Read the model definition and answer for the solid it produces. Units are mm, in the model's axes. Coordinates: 2 decimals unless noted, no trailing zeros. Write each loop counter-clockwise with the first axis right and the second up, starting at its lowest first coordinate (ties: lowest second). Pieces come first, ordered by that corner, then holes. Notation, with made-up numbers: (-34.75, -1) -> (-19.75, -1) arc R29 cw to (-19.75, 35) -> close; hole circle Ø5 at (-37, -23). An arc over 180 degrees is marked (long way). Use CSV: the item, a comma, the result in double quotes.
from build123d import *

# Parameters (mm, degrees)
ESQUISSE1_W                  = 1700
ESQUISSE1_H                  = 150
BOSS_EXTRU_1_DEPTH           = 25
ENL_V_MAT_EXTRU_1_DEPTH      = 1707.78791887
ENL_V_MAT_EXTRU_1_DEPTH_BACK = 1707.78791887
CHANFREIN2_SIZE              = 40
CHANFREIN3_SIZE              = 5


with BuildPart() as part:
    # Esquisse1 → Boss.-Extru.1 (new body)
    with BuildSketch(Plane.XY):
        with Locations((850, 75)):
            Rectangle(ESQUISSE1_W, ESQUISSE1_H)
    extrude(amount=BOSS_EXTRU_1_DEPTH)

    # Esquisse2 → Enlèv. mat.-Extru.1 (cut, two sides: drawn at the far end of the back side and taken through both)
    with BuildSketch(Plane(origin=(0, 150, 0), x_dir=(1, 0, 0), z_dir=(0, 1, 0)).offset(-ENL_V_MAT_EXTRU_1_DEPTH_BACK)):
        Polygon((100, 0), (101.227845609, -10), (61.227845609, -10), (62.455691218, 0), align=None)
        Polygon((1637.544308782, 0), (1638.772154391, -10), (1598.772154391, -10), (1600, 0), align=None)
        Polygon((868.772154391, 0), (831.227845609, 0), (830, -10), (870, -10), align=None)
    extrude(amount=ENL_V_MAT_EXTRU_1_DEPTH + ENL_V_MAT_EXTRU_1_DEPTH_BACK, mode=Mode.SUBTRACT)

    # Chanfrein2
    chanfrein2_edges = [part.edges().sort_by_distance(p)[0] for p in [
        (1700, 0, 12.5),
        (0, 0, 12.5),
    ]]
    chamfer(chanfrein2_edges, length=CHANFREIN2_SIZE)

    # Chanfrein3
    chanfrein3_edges = [part.edges().sort_by_distance(p)[0] for p in [
        (850, 150, 25),
        (0, 95, 25),
        (850, 0, 25),
        (1700, 95, 25),
        (1680, 20, 25),
        (20, 20, 25),
    ]]
    chamfer(chanfrein3_edges, length=CHANFREIN3_SIZE)


solid = part.part
1. A cutting plane is placed at A-A (y = 94.5). Give the vertices of the cut face in (x, z), and give its area (3 significant figures).
Solutions:
outline,"(0, 0) -> (62.46, 0) -> (61.23, 10) -> (101.23, 10) -> (100, 0) -> (831.23, 0) -> (830, 10) -> (870, 10) -> (868.77, 0) -> (1600, 0) -> (1598.77, 10) -> (1638.77, 10) -> (1637.54, 0) -> (1700, 0) -> (1700, 20) -> (1695, 25) -> (5, 25) -> (0, 20) -> close"
area,"41,300 mm^2"
2. This flat-tipped pin is pushed along its axis until it touches: pin 1 Ø1.5 at (x, z) = (447.5, 21.5) entering from -Y. Where does it stop, or does it pass through?
Solutions:
pin 1,"stops at y = 0.75"
3. A cutting plane is placed at B-B (y = 21). Give the vertices of the cut face in (x, z), and give its area (3 significant figures).
Solutions:
outline,"(19, 0) -> (62.46, 0) -> (61.23, 10) -> (101.23, 10) -> (100, 0) -> (831.23, 0) -> (830, 10) -> (870, 10) -> (868.77, 0) -> (1600, 0) -> (1598.77, 10) -> (1638.77, 10) -> (1637.54, 0) -> (1681, 0) -> (1681, 20) -> (1673.93, 25) -> (26.07, 25) -> (19, 20) -> close"
area,"40,400 mm^2"
4. Find the intervals of material crossed by line 1 along X through (y, z) = (65, 1.5); line 2 along X through (y, z) = (31, 5.75); line 3 along Z through (x, y) = (838, 50), in increasing order.
Solutions:
line 1,"x = 0 to 62.27, 100.18 to 831.04, 868.96 to 1599.82, 1637.73 to 1700"
line 2,"x = 9 to 61.75, 100.71 to 830.52, 869.48 to 1599.29, 1638.25 to 1691"
line 3,"z = 10 to 25"
